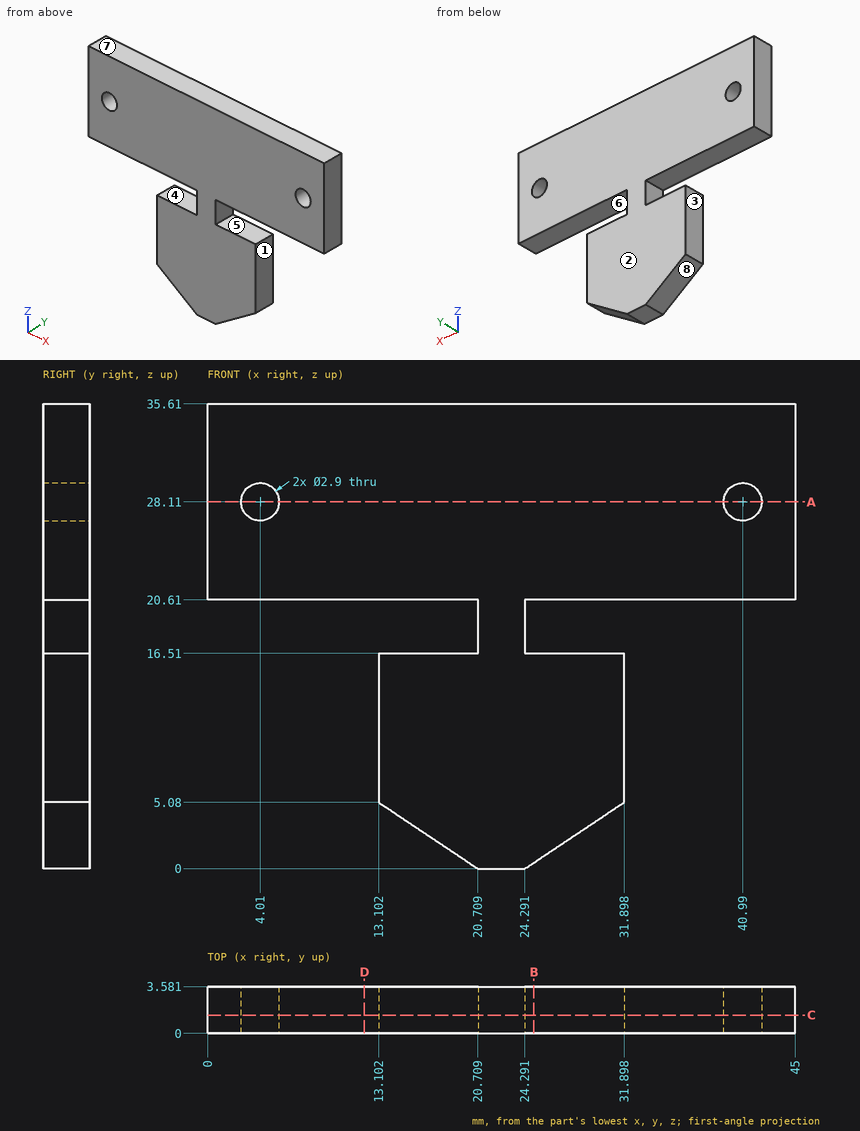
For this review, use the dimensioned drawing (mm, ordinates from the lowest corner) and the shaded views. A direction names the side the tool comes from. Round coordinates to 2 decimals unless told otherwise and drop trailing zeros. Order: outer loops, then holes, each group sorted by start corner. A loop starts at its lowest first (then second) coordinate and runs counter-clockwise, first axis right, second up. Notation, with made-up numbers: (56, 12) -> (114, 12) arc R13 ccw to (114, 37) -> close; hole circle Ø6 at (50.5, -2.5). An arc over 180 degrees is marked (long way). Write item = value, one per line. Start each with the question number.
Item 1: For the marked faces 1, 2, 3, 4 and 5, list the 3-axis set-ups (+Z, -Z, +X, -X, +Y, -Y) from which the entire face can be reached by the end or side of a thin tool; tool diameter is ignored.
Item 2: Consider section A-A on z = 28.11. Write out the cut boundary in (x, y).
Item 3: Mouldability with a two-part tool opening along Z and no side actions: class the marked faces 6, 7 and 8 as released by +Z, released by -Z, zero draft, split by the parting line, or undercut.
Item 4: Consider section C-C on y = 1.4. Write out the cut boundary in (x, z).
Item 5: Consider section D-D on x = 12. Write out the cut boundary in (y, z).
Item 6: Consider section B-B on x = 25. Write out the cut boundary in (y, z).
Item 7: For line 1 along X through (y, z) = (2.5, 28.11); line 2 along Z through (x, y) = (4.01, 2.5); line 3 along Z through (x, y) = (19, 2.5), list the stretches that pass through material, from the lowest coordinate up.
Item 8: Clearance check with flat-ended pins moving along their axes: pin 1 Ø1.8 at (x, y) = (35.5, 2.5) entering from -Z; pin 2 Ø1.8 at (y, z) = (2, 8.5) entering from -X; pin 3 Ø2.5 at (x, z) = (40.99, 28.11) entering from +Y; pin 4 Ø1.1 at (y, z) = (2.5, 18.5) entering from +X. State where each tip first meets the part, or that it passes through.
Conclusion:
q1.face_1 = -Z, +X, +Y, -Y
q1.face_2 = +Z, -Z, +X, -X, +Y
q1.face_3 = -Z, -X, +Y, -Y
q1.face_4 = -X, +Y, -Y
q1.face_5 = +X, +Y, -Y
q2.outline = (0, 0) -> (2.56, 0) -> (2.56, 3.58) -> (0, 3.58) -> close; (5.46, 0) -> (39.54, 0) -> (39.54, 3.58) -> (5.46, 3.58) -> close; (42.44, 0) -> (45, 0) -> (45, 3.58) -> (42.44, 3.58) -> close
q3.face_6 = undercut
q3.face_7 = released by +Z
q3.face_8 = released by -Z
q4.outline = (0, 20.61) -> (20.71, 20.61) -> (20.71, 16.51) -> (13.1, 16.51) -> (13.1, 5.08) -> (20.71, 0) -> (24.29, 0) -> (31.9, 5.08) -> (31.9, 16.51) -> (24.29, 16.51) -> (24.29, 20.61) -> (45, 20.61) -> (45, 35.61) -> (0, 35.61) -> close; hole circle Ø2.9 at (4.01, 28.11); hole circle Ø2.9 at (40.99, 28.11)
q5.outline = (0, 20.61) -> (3.58, 20.61) -> (3.58, 35.61) -> (0, 35.61) -> close
q6.outline = (0, 0.47) -> (3.58, 0.47) -> (3.58, 16.51) -> (0, 16.51) -> close; (0, 20.61) -> (3.58, 20.61) -> (3.58, 35.61) -> (0, 35.61) -> close
q7.line_1 = 0 to 2.56, 5.46 to 39.54, 42.44 to 45
q7.line_2 = 20.61 to 26.66, 29.56 to 35.61
q7.line_3 = 1.14 to 16.51, 20.61 to 35.61
q8.pin_1 = 20.61
q8.pin_2 = 13.1
q8.pin_3 = through
q8.pin_4 = 24.29
